Design review of the part built by this model. Coordinates are the model's own, in mm. A direction names the side the tool comes from. Coordinates: 2 decimals unless noted, no trailing zeros. Write each loop counter-clockwise with the first axis right and the second up, starting at its lowest first coordinate (ties: lowest second). Pieces come first, ordered by that corner, then holes.
Q1. Take a section at B-B, the plane z = 7. Write out the cut boundary in (x, y), plus the area to 3 significant figures.
Q2. The part is to be moulded in two halves that separate along Y. For faces 1 (the flat face through (0, 0, 8)), 2 (the flat face through (1.975, 1.119, 9.86)), 3 (the cylindrical face through (-1.5, 0.07, 13.98)), 4 (the flat face through (-2, 0, 20)), say which applies: released by +Y, released by -Y, zero draft, split by the parting line, or undercut.
Q3. For L1, parallel to Y at x = 0, z = 13.25; L2, parallel to X at y = -0.55, z = 13.25; L3, parallel to Z at x = 2, y = -0.85, list the stretches that pass through material, from the lowest coordinate up.
Q4. For faces 5 (the flat face through (0, 2, 0)), 6 (the flat face through (0, -2.27, 10)), list the 3-axis set-ups (+Z, -Z, +X, -X, +Y, -Y) from which the entire face can be reached by the end or side of a thin tool; tool diameter is ignored.
Q5. For pin 1 Ø1.5 at (x, y) = (0, -0.5) entering from +Z; pin 2 Ø1.5 at (x, z) = (2, -2) entering from +Y, all flat-tipped, find the tip position at first contact; note any pin that passes through.
Q6. Take a section at A-A, the plane z = 18. Write out the cut boundary in (x, y).
from build123d import *

# Parameters (mm, degrees)
BOSS_EXTRUDE1_DEPTH     = 20
SKETCH2_R               = 1.5
CUT_EXTRUDE1_DEPTH      = 1
CUT_EXTRUDE1_DEPTH_BACK = 12
CHAMFER1_SIZE           = 0.2
SKETCH4_R               = 1.5
BOSS_EXTRUDE2_DEPTH     = 6.5
CHAMFER2_SIZE           = 0.6


with BuildPart() as part:
    # Sketch1 → Boss-Extrude1 (new body)
    with BuildSketch(Plane.XY):
        Polygon((2.621170222, 0), (1.310585111, 2.27), (-1.310585111, 2.27), (-2.621170222, 0), (-1.310585111, -2.27), (1.310585111, -2.27), align=None)
    extrude(amount=BOSS_EXTRUDE1_DEPTH)

    # Sketch2 → Cut-Extrude1 (cut, two sides)
    with BuildSketch(Plane.XY.offset(20)) as cut_extrude1_sk:
        Circle(SKETCH2_R)
    extrude(amount=CUT_EXTRUDE1_DEPTH, mode=Mode.SUBTRACT)
    extrude(cut_extrude1_sk.sketch, amount=-CUT_EXTRUDE1_DEPTH_BACK, mode=Mode.SUBTRACT)

    # Sketch3 → Cut-Revolve1 (revolve, cut)
    with BuildSketch(Plane(origin=(0, 0, 0), x_dir=(1, 0, 0), z_dir=(0, 1, 0))):
        Polygon((-2.621170222, -20), (-2.271170222, -20), (-2.621170222, -19.8), align=None)
    revolve(axis=Axis((0, 0, 8), (0, 0, 1)), mode=Mode.SUBTRACT)

    # Chamfer1
    chamfer1_edges = [part.edges().sort_by_distance(p)[0] for p in [
        (-1.5, 0, 20),
    ]]
    chamfer(chamfer1_edges, length=CHAMFER1_SIZE)

    # Sketch4 → Boss-Extrude2 (add)
    with BuildSketch(Plane(origin=(0, 0, 0), x_dir=(-1, 0, 0), z_dir=(0, 0, -1))):
        Circle(SKETCH4_R)
    extrude(amount=BOSS_EXTRUDE2_DEPTH)

    # Chamfer2
    chamfer2_edges = [part.edges().sort_by_distance(p)[0] for p in [
        (1.5, 0, -6.5),
    ]]
    chamfer(chamfer2_edges, length=CHAMFER2_SIZE)


solid = part.part
Responses:
1. outline: (-2.62, 0) - (-1.31, -2.27) - (1.31, -2.27) - (2.62, 0) - (1.31, 2.27) - (-1.31, 2.27) - close
1. area: 17.9 mm2
2. face 1: undercut
2. face 2: released by +Y
2. face 3: undercut
2. face 4: zero draft
3. L1: y = -2.27 to -1.5, 1.5 to 2.27
3. L2: x = -2.3 to -1.4, 1.4 to 2.3
3. L3: z = 0 to 20
4. face 5: -Z
4. face 6: +Z, -Z, +X, -X, -Y
5. pin 1: stops at z = 8
5. pin 2: stops at y = 0.83
6. outline: (-2.62, 0) - (-1.31, -2.27) - (1.31, -2.27) - (2.62, 0) - (1.31, 2.27) - (-1.31, 2.27) - close; hole circle Ø3 at (0, 0)
